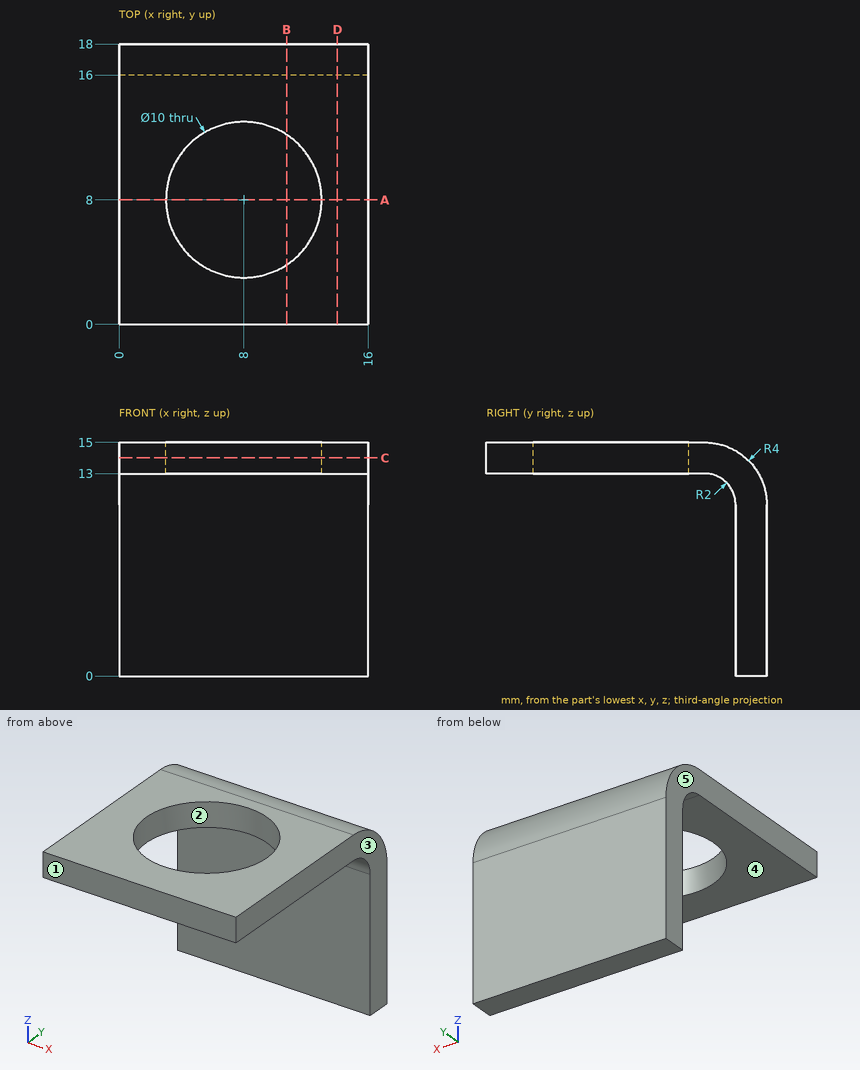
Source: three-view drawing plus pictorial views. Frame: mm from the lowest corner of the part. A direction names the side the tool comes from. Coordinates: 2 decimals unless noted, no trailing zeros. Loops run counter-clockwise (first coordinate to the right, second up) from the corner with the lowest first, then second, coordinate; pieces in that order, holes last. Notation, with made-up numbers: (23.5, 30) -> (73.5, 30) arc R12 ccw to (73.5, 34) -> close; hole circle Ø8 at (-36, 65). An arc over 180 degrees is marked (long way). One line per item, written item: value.
(1) Cut plane B-B (x = 10.75). Output: boundary loops of the cut face in (y, z), then the cut area to 3 significant figures.
Answer below:
outline: (0, 13) -> (3.82, 13) -> (3.82, 15) -> (0, 15) -> close; (12.18, 13) -> (14, 13) arc R2 cw to (16, 11) -> (16, 0) -> (18, 0) -> (18, 11) arc R4 ccw to (14, 15) -> (12.18, 15) -> close
area: 42.7 mm2
(2) Cut plane A-A (y = 8). Output: boundary loops of the cut face in (x, z).
Answer below:
outline: (0, 13) -> (3, 13) -> (3, 15) -> (0, 15) -> close; (13, 13) -> (16, 13) -> (16, 15) -> (13, 15) -> close
(3) Draft query along X for the marked faces 1, 2 and 3. Return one class per face: pulls with the +X half, pulls with the -X half, needs draft (parallel to the pull), parting line crosses it, or undercut.
Answer below:
face 1: needs draft
face 2: undercut
face 3: pulls with the +X half
(4) Pin query (flat end, axial travel): pin 1 Ø7 at (x, y) = (5, 9.5) entering from -Z; pin 2 Ø6 at (x, z) = (8, 2.5) entering from -Y. Return the tip coordinate at first contact, or that it passes through.
Answer below:
pin 1: stops at z = 13
pin 2: stops at y = 16
(5) Set-up query: the marked faces 4 and 5. Return all of +Z, -Z, +X, -X, +Y, -Y with unobstructed straight access to the full face (end or side cutting, diameter ignored); none if empty.
Answer below:
face 4: -Z, +X, -X, -Y
face 5: +Z, -Z, -X, +Y, -Y
(6) Cut plane D-D (x = 14). Output: boundary loops of the cut face in (y, z), then the cut area to 3 significant figures.
Answer below:
outline: (0, 13) -> (14, 13) arc R2 cw to (16, 11) -> (16, 0) -> (18, 0) -> (18, 11) arc R4 ccw to (14, 15) -> (0, 15) -> close
area: 59.4 mm2
(7) Cut plane C-C (z = 14). Output: boundary loops of the cut face in (x, y), then the cut area to 3 significant figures.
Answer below:
outline: (0, 0) -> (16, 0) -> (16, 16.65) -> (0, 16.65) -> close; hole circle Ø10 at (8, 8)
area: 188 mm2
(8) Ray query, line 1 along X through (y, z) = (8, 13.5); line 2 along Z through (x, y) = (7.75, 13.75); line 3 along Y through (x, z) = (10, 8.25). Return the intervals inside material, ascending.
Answer below:
line 1: x = 0 to 3, 13 to 16
line 2: z = 13 to 15
line 3: y = 16 to 18
